Here's how the part is built. I have some questions about the finished solid (model axes, mm). A direction names the side the tool comes from. Round coordinates to 2 decimals unless told otherwise and drop trailing zeros. Order: outer loops, then holes, each group sorted by start corner. A loop starts at its lowest first (then second) coordinate and runs counter-clockwise, first axis right, second up. Notation, with made-up numbers: M -31.5,-23.5 L 0.5,-23.5 A23 ccw 0.5,8.5 Z; hole C -2,12 d2. An arc over 180 degrees is marked long. Write item = value, one per line. Start each with the question number.
Item 1: I'm going to push flat-ended pins straight in: P1, Ø3, axis at x = -0.5, y = 0, coming from the -Z side; P2, Ø4, axis at x = -11, y = 9.5, coming from the -Z side. Where does each tip first touch, or does it pass through?
Item 2: We'd pull the mould along Y, two halves only. Please class faces 3 (the face through (8.73, -6.69, -0.88)), 4 (the face through (0, 0, 3.302)), 5 (the face through (0.69, -3.1, 0.73)), 6 (the face through (-12.809, 12.845, 16.279)): pulls with the +Y half, pulls with the -Y half, needs draft (parallel to the pull), parting line crosses it, or undercut.
Item 3: For faces 1 (the face through (12.845, 12.809, 16.279)), 2 (the face through (-10, 6, 0)), which set-ups out of +Z, -Z, +X, -X, +Y, -Y let a thin tool reach every point of the face, with its end or its side?
Item 4: I want a section at D-D, the plane x = -5. List the corners of the cut face in (y, z) for me.
Item 5: I want a section at A-A, the plane x = 0. List the corners of the cut face in (y, z) for me (3 decimals), plus the area to 3 significant figures.
Item 6: Please list where these lines run through material, in increasing order: L1, parallel to Y at x = 0, z = 1.7 (3 decimals); L2, parallel to Z at x = 7.5, y = -12.25; L3, parallel to Y at x = -12, z = 1.5.
Item 7: I want a section at B-B, the plane z = 30.5. List the corners of the cut face in (x, y) for me, plus the area to 3 significant figures.
```python
from build123d import *

# Parameters (mm, degrees)
SKETCH1_W           = 28.194
SKETCH1_H           = 28.194
BOSS_EXTRUDE1_DEPTH = 33.02
SKETCH3_R           = 10.9982
BOSS_EXTRUDE2_DEPTH = 1.778
SKETCH5_R           = 3.175
CUT_EXTRUDE1_DEPTH  = 5.08
CHAMFER1_SIZE       = 2.54


with BuildPart() as part:
    # Sketch1 → Boss-Extrude1 (new body)
    with BuildSketch(Plane.XY):
        Rectangle(SKETCH1_W, SKETCH1_H)
    extrude(amount=BOSS_EXTRUDE1_DEPTH)

    # Sketch3 → Boss-Extrude2 (add)
    with BuildSketch(Plane(origin=(0, 0, 0), x_dir=(-1, 0, 0), z_dir=(0, 0, -1))):
        Circle(SKETCH3_R)
    extrude(amount=BOSS_EXTRUDE2_DEPTH)

    # Sketch5 → Cut-Extrude1 (cut)
    with BuildSketch(Plane(origin=(0, 0, -1.778), x_dir=(-1, 0, 0), z_dir=(0, 0, -1))):
        Circle(SKETCH5_R)
    extrude(amount=-CUT_EXTRUDE1_DEPTH, mode=Mode.SUBTRACT)

    # Chamfer1
    chamfer1_edges = [part.edges().sort_by_distance(p)[0] for p in [
        (-14.097, 14.097, 16.51),
        (14.097, 14.097, 16.51),
        (14.097, -14.097, 16.51),
        (-14.097, -14.097, 16.51),
    ]]
    chamfer(chamfer1_edges, length=CHAMFER1_SIZE)


solid = part.part
```
Filled in:
q1.P1 = 3.3
q1.P2 = 0
q2.face_3 = parting line crosses it
q2.face_4 = undercut
q2.face_5 = undercut
q2.face_6 = pulls with the +Y half
q3.face_1 = +Z, -Z, +X, +Y
q3.face_2 = -Z
q4.outline = M -14.1,0 L -9.8,0 L -9.8,-1.78 L 9.8,-1.78 L 9.8,0 L 14.1,0 L 14.1,33.02 L -14.1,33.02 Z
q5.outline = M -14.097,0 L -10.998,0 L -10.998,-1.778 L -3.175,-1.778 L -3.175,3.302 L 3.175,3.302 L 3.175,-1.778 L 10.998,-1.778 L 10.998,0 L 14.097,0 L 14.097,33.02 L -14.097,33.02 Z
q5.area = 938 mm^2
q6.L1 = -14.097 to -3.175, 3.175 to 14.097
q6.L2 = 0 to 33.02
q6.L3 = -13.65 to 13.65
q7.outline = M -14.1,-11.56 L -11.56,-14.1 L 11.56,-14.1 L 14.1,-11.56 L 14.1,11.56 L 11.56,14.1 L -11.56,14.1 L -14.1,11.56 Z
q7.area = 782 mm^2
